Geometry: see drawing. Coordinates: mm, zero at the bounding-box minimum. Coordinates: 2 decimals unless noted, no trailing zeros. Write each loop counter-clockwise with the first axis right and the second up, starting at its lowest first coordinate (ties: lowest second). Pieces come first, ordered by that corner, then holes. Notation, with made-up numbers: (7, 34.25) - (64, 34.25) arc R17 cw to (64, 51.25) - close; hole circle Ø2 at (86.25, 37.25). An arc over 180 degrees is marked (long way). Use CSV: the item, a comma, the result in double quotes.
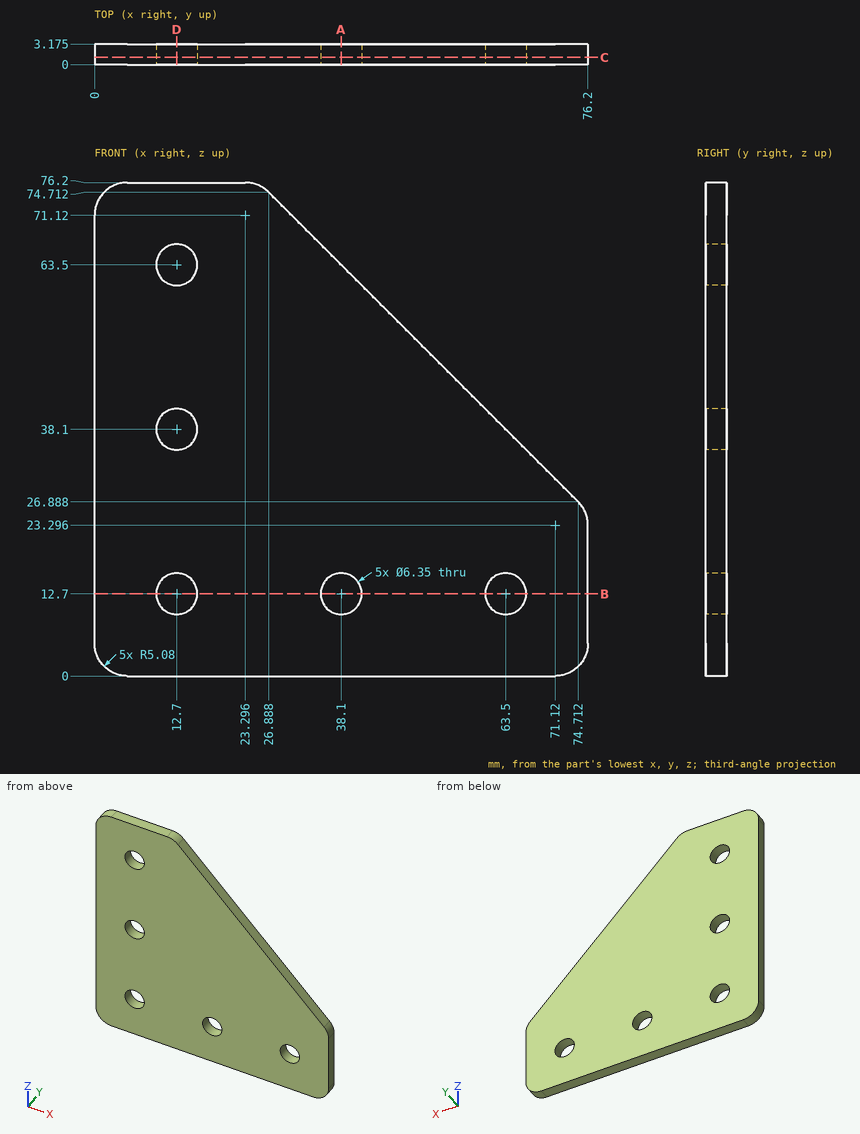
(1) Cut plane D-D on x = 12.7. Return loops of the section in (y, z) (3 decimals).
Check values:
outline,"(0, 0) - (3.175, 0) - (3.175, 9.525) - (0, 9.525) - close; (0, 15.875) - (3.175, 15.875) - (3.175, 34.925) - (0, 34.925) - close; (0, 41.275) - (3.175, 41.275) - (3.175, 60.325) - (0, 60.325) - close; (0, 66.675) - (3.175, 66.675) - (3.175, 76.2) - (0, 76.2) - close"
(2) Cut plane C-C on y = 1.1. State how many separate pieces and enclosed holes the cut face has, and give its area (3 significant figures).
Check values:
separate pieces,"1"
enclosed holes,"5"
area,"4,340 mm^2"
(3) Cut plane A-A on x = 38.1. Return loops of the section in (y, z) (3 decimals).
Check values:
outline,"(0, 0) - (3.175, 0) - (3.175, 9.525) - (0, 9.525) - close; (0, 15.875) - (3.175, 15.875) - (3.175, 63.5) - (0, 63.5) - close"
(4) Cut plane B-B on z = 12.7. Return loops of the section in (x, y) (3 decimals).
Check values:
outline,"(0, 0) - (9.525, 0) - (9.525, 3.175) - (0, 3.175) - close; (15.875, 0) - (34.925, 0) - (34.925, 3.175) - (15.875, 3.175) - close; (41.275, 0) - (60.325, 0) - (60.325, 3.175) - (41.275, 3.175) - close; (66.675, 0) - (76.2, 0) - (76.2, 3.175) - (66.675, 3.175) - close"
(5) Ray query, probe 1 along Z at (x, y) = (12.7, 0.6) (3 decimals); probe 2 along Z at (x, y) = (12, 2.05); probe 3 along Z at (x, y) = (38.1, 1.75) (1 decimal). Return the intervals inside material, ascending. Write a range as from..to.
Check values:
probe 1,"0..9.525, 15.875..34.925, 41.275..60.325, 66.675..76.2"
probe 2,"0..9.6, 15.8..35, 41.2..60.4, 66.6..76.2"
probe 3,"0..9.5, 15.9..63.5"
